from build123d import *

# Parameters (mm, degrees)
SKETCH2_W               = 27.8
SKETCH2_H               = 18
SKETCH2_R               = 6
BOSS_EXTRUDE1_DEPTH     = 15
SKETCH7_W               = 13.9
SKETCH7_H               = 15
SKETCH7_W_2             = 5.9
SKETCH7_H_2             = 5.9
BOSS_EXTRUDE3_DEPTH     = 1.8
SKETCH8_R               = 1.7
CUT_EXTRUDE3_DEPTH      = 29.464890655
FILLET4_R               = 0.5
FILLET4_OF_MIRROR1_R    = 0.5
MIRROR2_START           = -9
MIRROR2_OUTLINE_R       = 1.7
MIRROR2_DEPTH           = 18
MIRROR2_START_2         = 9
MIRROR2_2_OUTLINE_W     = 13.9
MIRROR2_2_OUTLINE_H     = 30
MIRROR2_2_DEPTH         = 1.8
FILLET3_R               = 2
BOSS_EXTRUDE4_DEPTH     = 1.7
CUT_EXTRUDE4_REACH      = 33.173
CUT_EXTRUDE4_END_RADIUS = 6
CUT_EXTRUDE4_START      = -1.5
SKETCH10_W              = 5.9
SKETCH10_H              = 5.9
FILLET5_R               = 0.5
SKETCH11_R              = 1.7
CUT_EXTRUDE5_DEPTH      = 29.604370348
FILLET5_OF_MIRROR3_R    = 0.5
CUT_EXTRUDE6_START      = -10.8
SKETCH12_W              = 2
SKETCH12_H              = 6
CUT_EXTRUDE6_DEPTH      = 10.8
SKETCH13_W              = 2
SKETCH13_H              = 6
CUT_EXTRUDE7_DEPTH      = 2.95
CUT_EXTRUDE8_REACH      = 35.384
CUT_EXTRUDE8_END_RADIUS = 6
SKETCH14_R              = 1.7


# Read off the part's stored shape, not the designer's step: Mirror2
with BuildPart() as part:
    # Sketch2 → Boss-Extrude1 (new, symmetric)
    with BuildSketch(Plane(origin=(0, 0, 0), x_dir=(1, 0, 0), z_dir=(0, 1, 0))):
        Rectangle(SKETCH2_W, SKETCH2_H)
        with Locations(Location((0, 0, 0), (0, 0, 270))):
            Circle(SKETCH2_R, mode=Mode.SUBTRACT)
    extrude(amount=BOSS_EXTRUDE1_DEPTH, both=True)

    # Sketch7 → Boss-Extrude3 (add)
    with BuildSketch(Plane.XY.offset(9)):
        with Locations((-6.95, 7.5)):
            Rectangle(SKETCH7_W, SKETCH7_H)
        with Locations((-9.2, 10.3)):
            Rectangle(SKETCH7_W_2, SKETCH7_H_2, mode=Mode.SUBTRACT)
    boss_extrude3 = extrude(amount=BOSS_EXTRUDE3_DEPTH)

    # Sketch8 → Cut-Extrude3 (cut, through all)
    with BuildSketch(Plane.XY.offset(10.8)):
        with Locations((-9.2, 10.3)):
            Circle(SKETCH8_R)
    cut_extrude3 = extrude(amount=-CUT_EXTRUDE3_DEPTH, mode=Mode.SUBTRACT)

    # Fillet4
    fillet4_edges = [part.edges().sort_by_distance(p)[0] for p in [
        (-6.25, 13.25, 9.9),
        (-12.15, 13.25, 9.9),
        (-12.15, 7.35, 9.9),
        (-6.25, 7.35, 9.9),
    ]]
    fillet(fillet4_edges, radius=FILLET4_R)

    # Mirror1: Boss-Extrude3, Cut-Extrude3 across plane
    add(boss_extrude3.mirror(Plane.ZX))
    add(cut_extrude3.mirror(Plane.ZX), mode=Mode.SUBTRACT)

    # Fillet4 of Mirror1
    fillet4_of_mirror1_edges = [part.edges().sort_by_distance(p)[0] for p in [
        (-6.25, -13.25, 9.9),
        (-12.15, -13.25, 9.9),
        (-12.15, -7.35, 9.9),
        (-6.25, -7.35, 9.9),
    ]]
    fillet(fillet4_of_mirror1_edges, radius=FILLET4_OF_MIRROR1_R)

    # Mirror2 outline → Mirror2 (cut)
    with BuildSketch(Plane.XY.offset(MIRROR2_START)):
        with Locations((9.2, -10.3)):
            Circle(MIRROR2_OUTLINE_R)
        with Locations((9.2, 10.3)):
            Circle(MIRROR2_OUTLINE_R)
    extrude(amount=MIRROR2_DEPTH, mode=Mode.SUBTRACT)

    # Mirror2 2 outline → Mirror2 2 (add)
    with BuildSketch(Plane.XY.offset(MIRROR2_START_2)):
        with Locations((6.95, 0)):
            Rectangle(MIRROR2_2_OUTLINE_W, MIRROR2_2_OUTLINE_H)
        with BuildLine():
            ThreePointArc((6.25, -7.85), (6.396446609, -7.496446609), (6.75, -7.35))
            Line((6.75, -7.35), (11.65, -7.35))
            ThreePointArc((11.65, -7.35), (12.003553391, -7.496446609), (12.15, -7.85))
            Line((12.15, -7.85), (12.15, -12.75))
            ThreePointArc((12.15, -12.75), (12.003553391, -13.103553391), (11.65, -13.25))
            Line((11.65, -13.25), (6.75, -13.25))
            ThreePointArc((6.75, -13.25), (6.396446609, -13.103553391), (6.25, -12.75))
            Line((6.25, -12.75), (6.25, -7.85))
        make_face(mode=Mode.SUBTRACT)
        with BuildLine():
            Line((6.75, 13.25), (11.65, 13.25))
            ThreePointArc((11.65, 13.25), (12.003553391, 13.103553391), (12.15, 12.75))
            Line((12.15, 12.75), (12.15, 7.85))
            ThreePointArc((12.15, 7.85), (12.003553391, 7.496446609), (11.65, 7.35))
            Line((11.65, 7.35), (6.75, 7.35))
            ThreePointArc((6.75, 7.35), (6.396446609, 7.496446609), (6.25, 7.85))
            Line((6.25, 7.85), (6.25, 12.75))
            ThreePointArc((6.25, 12.75), (6.396446609, 13.103553391), (6.75, 13.25))
        make_face(mode=Mode.SUBTRACT)
    extrude(amount=MIRROR2_2_DEPTH)

    # Fillet3
    fillet3_edges = [part.edges().sort_by_distance(p)[0] for p in [
        (-13.9, 15, 0.9),
        (13.9, 15, 0.9),
        (-13.9, -15, 0.9),
        (13.9, -15, 0.9),
    ]]
    fillet(fillet3_edges, radius=FILLET3_R)

    # Sketch9 → Boss-Extrude4 (add)
    with BuildSketch(Plane(origin=(0, 0, -9), x_dir=(-1, 0, 0), z_dir=(0, 0, -1))):
        Polygon((-3.1, 15), (3.1, 15), (3.1, 6), (4.1, 6), (4.1, -15), (-4.1, -15), (-4.1, 6), (-3.1, 6), align=None)
    extrude(amount=BOSS_EXTRUDE4_DEPTH)

    # Cut-Extrude4: up to this cylinder (the profile starts outside it)
    cut_extrude4_end = Plane(origin=(0, 10.3, 0), z_dir=(0, -1, 0)) * Cylinder(CUT_EXTRUDE4_END_RADIUS, 79.346, mode=Mode.PRIVATE)
    # Sketch10 → Cut-Extrude4 (cut, up to the surface)
    with BuildSketch(Plane.XY.offset(10.8).offset(CUT_EXTRUDE4_START), mode=Mode.PRIVATE) as cut_extrude4_sk1:
        with Locations((0, 10.3)):
            Rectangle(SKETCH10_W, SKETCH10_H)
    cut_extrude4_tool1 = extrude(cut_extrude4_sk1.sketch, amount=-CUT_EXTRUDE4_REACH, mode=Mode.PRIVATE) - cut_extrude4_end
    cut_extrude4 = cut_extrude4_tool1.solids().sort_by_distance((0, 10.3, 9.3))[0]
    add(cut_extrude4, mode=Mode.SUBTRACT)

    # Fillet5
    fillet5_edges = [part.edges().sort_by_distance(p)[0] for p in [
        (2.95, 13.25, 7.262350474),
        (2.95, 7.35, 7.262350474),
        (-2.95, 7.35, 7.262350474),
        (-2.95, 13.25, 7.262350474),
    ]]
    fillet(fillet5_edges, radius=FILLET5_R)

    # Sketch11 → Cut-Extrude5 (cut, through all)
    with BuildSketch(Plane(origin=(0, 0, 9.3), x_dir=(-1, 0, 0), z_dir=(0, 0, -1))):
        with Locations((0, 10.3)):
            Circle(SKETCH11_R)
    cut_extrude5 = extrude(amount=-CUT_EXTRUDE5_DEPTH, mode=Mode.SUBTRACT)

    # Mirror3: Cut-Extrude4, Cut-Extrude5 across plane
    add(cut_extrude4.mirror(Plane.ZX), mode=Mode.SUBTRACT)
    add(cut_extrude5.mirror(Plane.ZX), mode=Mode.SUBTRACT)

    # Fillet5 of Mirror3
    fillet5_of_mirror3_edges = [part.edges().sort_by_distance(p)[0] for p in [
        (2.95, -13.25, 7.262350474),
        (2.95, -7.35, 7.262350474),
        (-2.95, -7.35, 7.262350474),
        (-2.95, -13.25, 7.262350474),
    ]]
    fillet(fillet5_of_mirror3_edges, radius=FILLET5_OF_MIRROR3_R)

    # Sketch12 → Cut-Extrude6 (cut)
    with BuildSketch(Plane.XY.offset(10.8).offset(CUT_EXTRUDE6_START)):
        with Locations((-9.9, 0)):
            Rectangle(SKETCH12_W, SKETCH12_H)
    cut_extrude6 = extrude(amount=CUT_EXTRUDE6_DEPTH, mode=Mode.SUBTRACT)

    # Sketch13 → Cut-Extrude7 (cut)
    with BuildSketch(Plane.XY):
        with Locations((-9.9, 0)):
            Rectangle(SKETCH13_W, SKETCH13_H)
    cut_extrude7 = extrude(amount=-CUT_EXTRUDE7_DEPTH, mode=Mode.SUBTRACT)

    # Cut-Extrude8: up to this cylinder (the profile starts outside it)
    cut_extrude8_end = Plane(origin=(0, 0, 0), z_dir=(0, -1, 0)) * Cylinder(CUT_EXTRUDE8_END_RADIUS, 83.768, mode=Mode.PRIVATE)
    # Sketch14 → Cut-Extrude8 (cut, up to the surface)
    with BuildSketch(Plane.ZY.offset(13.9), mode=Mode.PRIVATE) as cut_extrude8_sk1:
        Circle(SKETCH14_R)
    cut_extrude8_tool1 = extrude(cut_extrude8_sk1.sketch, amount=-CUT_EXTRUDE8_REACH, mode=Mode.PRIVATE) - cut_extrude8_end
    cut_extrude8 = cut_extrude8_tool1.solids().sort_by_distance((-13.9, 0, 0))[0]
    add(cut_extrude8, mode=Mode.SUBTRACT)

    # Mirror4: Cut-Extrude6, Cut-Extrude7, Cut-Extrude8 across plane
    add(cut_extrude6.mirror(Plane(origin=(0, 0, 0), x_dir=(0, 0, 1), z_dir=(1, 0, 0))), mode=Mode.SUBTRACT)
    add(cut_extrude7.mirror(Plane(origin=(0, 0, 0), x_dir=(0, 0, 1), z_dir=(1, 0, 0))), mode=Mode.SUBTRACT)
    add(cut_extrude8.mirror(Plane(origin=(0, 0, 0), x_dir=(0, 0, 1), z_dir=(1, 0, 0))), mode=Mode.SUBTRACT)


solid = part.part
The listing builds one solid part. Answer for the finished solid, in the listing's coordinates (mm). A direction names the side the tool comes from. Give positions to 0.01 mm unless a question says otherwise; leave off trailing zeros. Loops run counter-clockwise (first coordinate to the right, second up) from the corner with the lowest first, then second, coordinate; pieces in that order, holes last.
Item 1: Determine the mould class of faces 1 (the flat face through (0, 13.25, 7)), 2 (the flat face through (-9, 0, -9)), 3 (the cylindrical face through (-13.3, -14.43, 1.04)) for opening direction Y: +Y half, -Y half, draft (parallel to the pull), parting line (faces both ways), or undercut.
Derived:
face 1: undercut
face 2: draft
face 3: -Y half
Item 2: A tool of negligible diameter and unlimited length cuts with its end or side. For faces 4 (the flat face through (9, -7.35, 10)), 5 (the flat face through (2.95, 10, 7)), 6 (the flat face through (-4.1, -4, -10)), from which of +Z, -Z, +X, -X, +Y, -Y can it reach the whole face along a straight path? Write none if from no direction.
Derived:
face 4: +Z
face 5: none
face 6: -Z, -X, +Y, -Y
Item 3: A cutting plane is placed at A-A (y = -10.3). Give the number of separate pieces and of enclosed holes in the cut face, then the cut area to 3 significant figures.
Derived:
separate pieces: 3
enclosed holes: 0
area: 282 mm2
Item 4: A cutting plane is placed at B-B (z = 2.25). Give the vertices of the cut face in (x, y), then the cut area to 3 significant figures.
Derived:
outline: (-13.9, -13) arc R2 ccw to (-11.9, -15) - (-5.56, -15) - (-5.56, 15) - (-11.9, 15) arc R2 ccw to (-13.9, 13) - close; (5.56, -15) - (11.9, -15) arc R2 ccw to (13.9, -13) - (13.9, 13) arc R2 ccw to (11.9, 15) - (5.56, 15) - close; hole circle Ø3.4 at (-9.2, -10.3); hole (-10.9, -3) - (-8.9, -3) - (-8.9, 3) - (-10.9, 3) - close; hole circle Ø3.4 at (-9.2, 10.3); hole circle Ø3.4 at (9.2, -10.3); hole circle Ø3.4 at (9.2, 10.3); hole (8.9, -3) - (10.9, -3) - (10.9, 3) - (8.9, 3) - close
area: 437 mm2
Item 5: Find the intervals of material crossed by line 1 along Y through (x, z) = (0, 9.8); line 2 along X through (y, z) = (-4.5, 0); line 3 along Y through (x, z) = (9.25, 0), in increasing order.
Derived:
line 1: y = -15 to -12, -8.6 to 8.6, 12 to 15
line 2: x = -13.9 to -6, 6 to 13.9
line 3: y = -15 to -12, -8.6 to -3, 3 to 8.6, 12 to 15
Item 6: Each of these flat-tipped pins is pushed along its axis until it touches: pin 1 Ø3 at (x, y) = (9.5, -11) entering from +Z; pin 2 Ø1.9 at (y, z) = (9.5, -10) entering from -X. Where does it stop, or does it pass through?
Derived:
pin 1: stops at z = 9
pin 2: stops at x = -3.1
